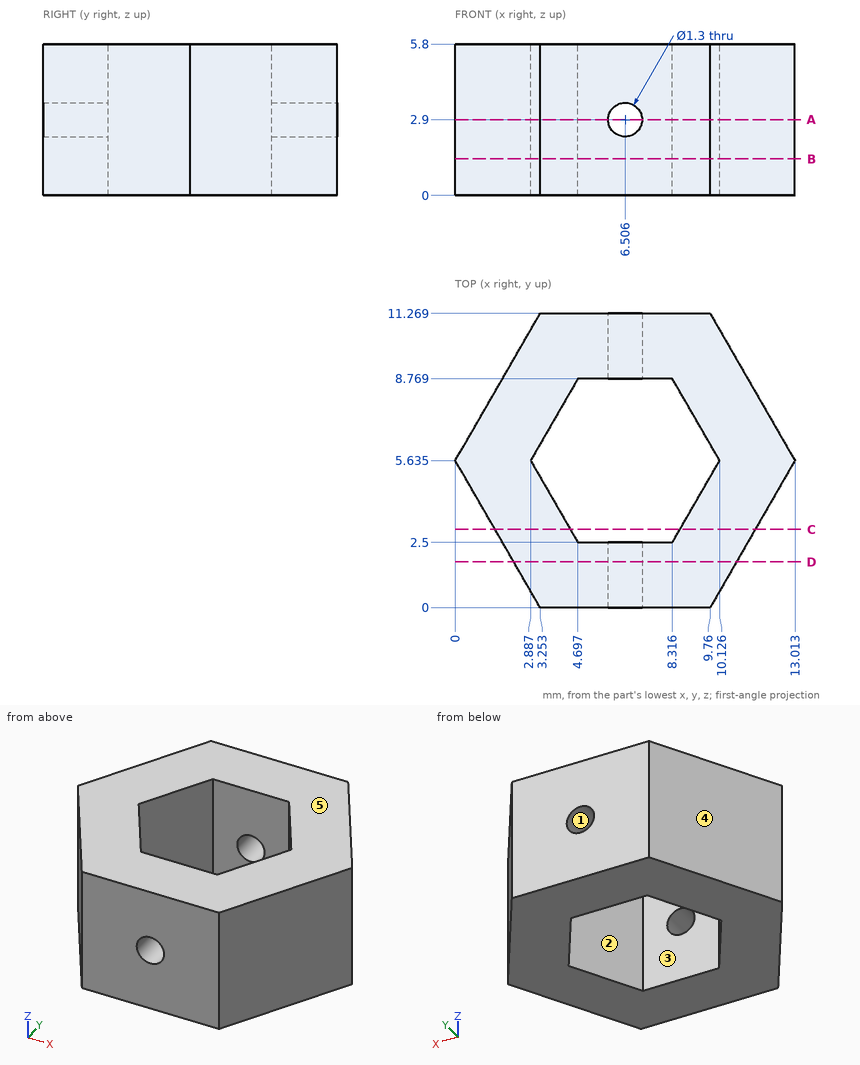
Verification items for this drawing (mm, ordinates from the low corner). A direction names the side the tool comes from. Give positions to 0.01 mm unless a question says otherwise; leave off trailing zeros. Loops run counter-clockwise (first coordinate to the right, second up) from the corner with the lowest first, then second, coordinate; pieces in that order, holes last. Notation, with made-up numbers: M 59.25,-8 L 109.25,-8 A25 cw 109.25,9 Z; hole C -30.75,68 d11. An arc over 180 degrees is marked long. Return JSON: item names as keys, results as strings. Group by question number.
1. Cross-section at C-C on y = 3. Record the boundary of the cut face in (x, z) (1 decimal).
2. Tool access check on the marked faces 1 and 2. Record the directions out of +Z, -Z, +X, -X, +Y, -Y that give a thin tool (end or side, any length) a straight path to the whole face; none if there is none.
3. Go/stop test with a flat-tipped pin: pin 1 (1.5 mm diameter, centred on y = 7, z = 2, fed in from -X) (1 decimal). Record where the tip stops, or that it passes through.
4. Cross-section at A-A on z = 2.9. Record the boundary of the cut face in (x, y) (1 decimal).
5. Cross-section at D-D on y = 1.75. Record the boundary of the cut face in (x, z).
6. Thickness scan on L1, parallel to Y at x = 8, z = 4.6; L2, parallel to Z at x = 6.75, y = 9.75; L3, parallel to X at y = 1.75, z = 2.9 (1 decimal). Record the ranges inside material, lowest first.
7. Mould release check, pull along Y, two halves, no side actions. Record for the marked faces 3, 4 and 5: released by +Y, released by -Y, zero draft, split by the parting line, or undercut.
8. Cross-section at B-B on z = 1.4. Record the boundary of the cut face in (x, y) (1 decimal).
Return value:
{
 "1": {"outline": "M 1.5,0 L 4.4,0 L 4.4,5.8 L 1.5,5.8 Z; M 8.6,0 L 11.5,0 L 11.5,5.8 L 8.6,5.8 Z"},
 "2": {"face 1": "+Y, -Y", "face 2": "+Z, -Z"},
 "3": {"pin 1": "x = 0.4"},
 "4": {"outline": "M 0,5.6 L 3.3,0 L 5.9,0 L 5.9,2.5 L 4.7,2.5 L 2.9,5.6 L 4.7,8.8 L 5.9,8.8 L 5.9,11.3 L 3.3,11.3 Z; M 7.2,0 L 9.8,0 L 13,5.6 L 9.8,11.3 L 7.2,11.3 L 7.2,8.8 L 8.3,8.8 L 10.1,5.6 L 8.3,2.5 L 7.2,2.5 Z"},
 "5": {"outline": "M 2.24,0 L 10.77,0 L 10.77,5.8 L 2.24,5.8 Z; hole C 6.51,2.9 d1.3"},
 "6": {"L1": "0 to 2.5, 8.77 to 11.27", "L2": "0 to 2.3, 3.5 to 5.8", "L3": "2.2 to 5.9, 7.2 to 10.8"},
 "7": {"face 3": "undercut", "face 4": "released by +Y", "face 5": "zero draft"},
 "8": {"outline": "M 0,5.6 L 3.3,0 L 9.8,0 L 13,5.6 L 9.8,11.3 L 3.3,11.3 Z; hole M 2.9,5.6 L 4.7,2.5 L 8.3,2.5 L 10.1,5.6 L 8.3,8.8 L 4.7,8.8 Z"}
}
